Autodesk Fusion 360 part; units mm, degrees
sketch "Skizze1" plane through (0, 0, 0) normal (0, 0, 1) x (1, 0, 0)
  line L0 (60, 0) -> (310, 0)
  line L1 (370, 60) -> (370, 310)
  line L2 (310, 370) -> (60, 370)
  line L3 (0, 310) -> (0, 60)
  line L4 (120, 60) -> (250, 60)
  line L5 (310, 120) -> (310, 250)
  line L6 (250, 310) -> (120, 310)
  line L7 (60, 250) -> (60, 120)
  arc A0 (120, 310) -> (60, 250) centre (120, 250) ccw
  arc A1 (310, 250) -> (250, 310) centre (250, 250) ccw
  arc A2 (250, 60) -> (310, 120) centre (250, 120) ccw
  arc A3 (60, 120) -> (120, 60) centre (120, 120) ccw
  arc A4 (310, 0) -> (370, 60) centre (310, 60) ccw
  arc A5 (0, 60) -> (60, 0) centre (60, 60) ccw
  arc A6 (60, 370) -> (0, 310) centre (60, 310) ccw
  arc A7 (370, 310) -> (310, 370) centre (310, 310) ccw
  line L8 (368.5, 60) -> (368.5, 310)
  arc A8 (368.5, 310) -> (310, 368.5) centre (310, 310) ccw
  line L9 (310, 368.5) -> (60, 368.5)
  arc A9 (60, 368.5) -> (1.5, 310) centre (60, 310) ccw
  line L10 (1.5, 310) -> (1.5, 60)
  arc A10 (1.5, 60) -> (60, 1.5) centre (60, 60) ccw
  line L11 (60, 1.5) -> (310, 1.5)
  arc A11 (310, 1.5) -> (368.5, 60) centre (310, 60) ccw
  line L12 (120, 58.5) -> (250, 58.5)
  arc A12 (250, 58.5) -> (311.5, 120) centre (250, 120) ccw
  line L13 (311.5, 120) -> (311.5, 250)
  arc A13 (311.5, 250) -> (250, 311.5) centre (250, 250) ccw
  line L14 (250, 311.5) -> (120, 311.5)
  arc A14 (120, 311.5) -> (58.5, 250) centre (120, 250) ccw
  line L15 (58.5, 250) -> (58.5, 120)
  arc A15 (58.5, 120) -> (120, 58.5) centre (120, 120) ccw
  line L16 (105, 5) -> (265, 5)
  line L17 (265, 5) -> (265, 55)
  line L18 (265, 55) -> (105, 55)
  line L19 (105, 55) -> (105, 5)
  line L20 (310, 60) -> (325, 60)
  line L21 (325, 60) -> (325, 45)
  line L22 (325, 45) -> (310, 45)
  line L23 (310, 45) -> (310, 60)
  line L24 (312.5, 57.5) -> (322.5, 57.5)
  line L25 (322.5, 57.5) -> (322.5, 47.5)
  line L26 (322.5, 47.5) -> (312.5, 47.5)
  line L27 (312.5, 47.5) -> (312.5, 57.5)
  line L28 (310, 310) -> (325, 310)
  line L29 (325, 310) -> (325, 325)
  line L30 (325, 325) -> (310, 325)
  line L31 (310, 325) -> (310, 310)
  line L32 (60, 310) -> (45, 310)
  line L33 (45, 310) -> (45, 325)
  line L34 (45, 325) -> (60, 325)
  line L35 (60, 325) -> (60, 310)
  line L36 (57.5, 312.5) -> (47.5, 312.5)
  line L37 (47.5, 312.5) -> (47.5, 322.5)
  line L38 (47.5, 322.5) -> (57.5, 322.5)
  line L39 (57.5, 322.5) -> (57.5, 312.5)
  line L40 (322.5, 312.5) -> (322.5, 322.5)
  line L41 (322.5, 322.5) -> (312.5, 322.5)
  line L42 (312.5, 322.5) -> (312.5, 312.5)
  line L43 (312.5, 312.5) -> (322.5, 312.5)
  line L44 (60, 60) -> (45, 60)
  line L45 (45, 60) -> (45, 45)
  line L46 (45, 45) -> (60, 45)
  line L47 (60, 45) -> (60, 60)
  line L48 (47.5, 47.5) -> (57.5, 47.5)
  line L49 (57.5, 47.5) -> (57.5, 57.5)
  line L50 (57.5, 57.5) -> (47.5, 57.5)
  line L51 (47.5, 57.5) -> (47.5, 47.5)
  circle A16 centre (110, 50) radius 5
  circle A17 centre (110, 10) radius 5
  circle A18 centre (260, 50) radius 5
  circle A19 centre (260, 10) radius 5
  point P0 (370, 0)
  point P1 (0, 370)
  dimension "d3" = 370
  dimension "d4" = 370
  dimension "d6" = 60
  dimension "d7" = -1.5
  dimension "d8" = 1.5
  dimension "d11" = 160
  dimension "d12" = 50
  dimension "d13" = 15
  dimension "d14" = 15
  dimension "d15" = 2.5
  dimension "d16" = 15
  dimension "d17" = 15
  dimension "d18" = 15
  dimension "d19" = 15
  dimension "d20" = 2.5
  dimension "d21" = -2.5
  dimension "d22" = 15
  dimension "d23" = 15
  dimension "d24" = -2.5
  dimension "d35" = 10
  dimension "d36" = 10
  dimension "d37" = 10
  dimension "d38" = 10
extrude "Extrusion1" add sketch "Skizze1" along normal blind 2 contours L16 L19 A17 | L16 L17 L18 L19 A16 A17 A18 A19 | A17 | L16 L17 A19 | A19 | L18 L19 A16 | A16 | L17 L18 A18 | A18 | L20 L21 L22 L23 | L24 L25 L26 L27 | L28 L29 L30 L31 | L32 L33 L34 L35 | L36 L37 L38 L39 | L40 L41 L42 L43 | L44 L45 L46 L47 | L48 L49 L50 L51 makes body 1 at (50, 55, 0) makes body 2 at (315, 55, 0) makes body 3 at (55, 315, 0) makes body 4 at (158.3333, 38.3333, 0) makes body 5 at (315, 320, 0)
extrude "Extrusion2" add sketch "Skizze1" along normal blind 2 contours L8 A8 L9 A9 L10 A10 L11 A11 bodies 1 2 3 4 5
extrude "Extrusion3" add sketch "Skizze1" along normal blind 20 contours L0 L1 L2 L3 A4 A5 A6 A7 | L12 A12 L13 A13 L14 A14 L15 A15 bodies 1
extrude "Extrusion4" add sketch "Skizze1" along normal blind 2 separate body contours L24 L25 L26 L27 | L36 L37 L38 L39 | L40 L41 L42 L43 | L48 L49 L50 L51 makes body 6 at (319.1667, 315.8333, 0) makes body 7 at (50.8333, 54.1667, 0) makes body 8 at (54.1667, 315.8333, 0) makes body 9 at (315.8333, 54.1667, 0)
extrude "Extrusion5" add sketch "Skizze1" along normal blind 20 contours L20 L21 L22 L23 | L28 L29 L30 L31 | L32 L33 L34 L35 | L44 L45 L46 L47 bodies 1 6 7 8 9
The listing builds one solid part. Answer for the finished solid, in the listing's coordinates (mm). A direction names the side the tool comes from. Round coordinates to 2 decimals unless told otherwise and drop trailing zeros. Order: outer loops, then holes, each group sorted by start corner. A loop starts at its lowest first (then second) coordinate and runs counter-clockwise, first axis right, second up. Notation, with made-up numbers: (-6.5, 63.25) -> (36.5, 63.25) arc R18 ccw to (36.5, 96.25) -> close; hole circle Ø9 at (64.5, 87.5). An arc over 180 degrees is marked (long way). Answer as CSV lines item,"result". Start each with the question number.
(1) Flat-ended cylindrical pins translate along their axes: pin 1 Ø5 at (x, z) = (50.5, 9.5) entering from +Y; pin 2 Ø7.5 at (x, z) = (315.5, 15.5) entering from +Y; pin 3 Ø5 at (x, z) = (318.5, 7) entering from +Y. Find the tip coordinate at first contact, or state that the pin passes through.
(2) A tool of negligible diameter and unlimited length cuts with its end or side. For faces 5 (the face through (351.818, 19.092, 10.874)), 6 (the face through (352.89, 18.04, 9.86)), 7 (the face through (184, 60, 10)), from which of +Z, -Z, +X, -X, +Y, -Y can it reach the whole face along a straight path? Write none if from no direction.
(3) The part is cut by section D-D (y = 340). Determine the outline of the cut face in (x, z), then the cut area to 3 significant figures.
(4) Find the intervals of material crossed by probe 1 along X at (y, z) = (250, 5.5); probe 2 along X at (y, z) = (94, 2.25), in increasing order. Write a range as from..to.
(5) The part is cut by section A-A (y = 209.5). Determine the outline of the cut face in (x, z), then the cut area to 3 significant figures.
(6) The part is cut by section C-C (z = 12.75). Count the separate pieces of the cut face and the enclosed holes in it, then the cut area to 3 significant figures.
(7) For a pull along Y with two mould halves and no side action, classify faces 1 (the face through (76.99, 76.04, 10.87)), 2 (the face through (317, 58, 20)), 3 (the face through (18.04, 17.11, 9.86)), 4 (the face through (318, 47.5, 11)) as +Y half, -Y half, draft (parallel to the pull), parting line (faces both ways), or undercut.
Evaluation:
1,pin 1,"y = 369.59"
1,pin 2,"y = 369.97"
1,pin 3,"y = 369.7"
2,face 5,"+Z"
2,face 6,"+Z, -Z, +X, -Y"
2,face 7,"+Z, -Z"
3,outline,"(8.04, 0) -> (361.96, 0) -> (361.96, 20) -> (360.22, 20) -> (360.22, 2) -> (9.78, 2) -> (9.78, 20) -> (8.04, 20) -> close"
3,area,"770 mm²"
4,probe 1,"0..1.5, 58.5..60, 310..311.5, 368.5..370"
4,probe 2,"0..1.5, 64.27..65.93, 304.07..305.73, 368.5..370"
5,outline,"(0, 0) -> (60, 0) -> (60, 20) -> (58.5, 20) -> (58.5, 2) -> (1.5, 2) -> (1.5, 20) -> (0, 20) -> close; (310, 0) -> (370, 0) -> (370, 20) -> (368.5, 20) -> (368.5, 2) -> (311.5, 2) -> (311.5, 20) -> (310, 20) -> close"
5,area,"348 mm²"
6,separate pieces,"6"
6,enclosed holes,"6"
6,area,"3,910 mm²"
7,face 1,"undercut"
7,face 2,"draft"
7,face 3,"-Y half"
7,face 4,"undercut"
